The listing builds one solid part. Answer for the finished solid, in the listing's coordinates (mm). Coordinates: 2 decimals unless noted, no trailing zeros. Loops run counter-clockwise (first coordinate to the right, second up) from the corner with the lowest first, then second, coordinate; pieces in that order, holes last. Notation, with made-up numbers: (3, -9.5) - (15, -9.5) arc R8 cw to (15, -2.5) - close; hole circle Ø6 at (-22.5, 29). An arc over 180 degrees is marked (long way). One line per question, with ' | ' between items.
from build123d import *

# Parameters (mm, degrees)
F1_DEPTH = 254
F2_R     = 5.08
F3_R     = 11.0334695749
F3_R_2   = 10.3236193182
F3_R_3   = 10.3446634655
F4_DEPTH = 461.264


# Not quite as in the source:
# - the program builds the solid bodies; features that only make, move or delete a surface that nothing else refers to are left out


with BuildPart() as f1:
    # F0 (on Front) → F1 (new body)
    with BuildSketch(Plane.XZ):
        with BuildLine():
            ThreePointArc((-30.4000387615, -20.3651585358), (-24.0059784619, -10.8970905515), (-21.758691331, 0.3046065976))
            ThreePointArc((-21.758691331, 0.3046065976), (-23.9392938004, 11.3454431448), (-30.1536347581, 20.7282500411))
            ThreePointArc((-30.1536347581, 20.7282500411), (-36.5903525714, 0.2194028111), (-30.4000387615, -20.3651585358))
        make_face()
        with BuildLine():
            ThreePointArc((-30.1536347581, 20.7282500411), (-23.9392938004, 11.3454431448), (-21.758691331, 0.3046065976))
            ThreePointArc((-21.758691331, 0.3046065976), (-24.0059784619, -10.8970905515), (-30.4000387615, -20.3651585358))
            ThreePointArc((-30.4000387615, -20.3651585358), (-0.593995823, -36.5861887582), (29.7229129207, -21.3412859593))
            ThreePointArc((29.7229129207, -21.3412859593), (20.8050989976, 0), (29.7229129207, 21.3412859593))
            ThreePointArc((29.7229129207, 21.3412859593), (-0.3746112446, 36.5890927095), (-30.1536347581, 20.7282500411))
        make_face()
        with BuildLine():
            ThreePointArc((-30.4000387615, -20.3651585358), (-36.5903525714, 0.2194028111), (-30.1536347581, 20.7282500411))
            ThreePointArc((-30.1536347581, 20.7282500411), (-79.8407866027, 0.4787407551), (-30.4000387615, -20.3651585358))
        make_face()
        with BuildLine():
            ThreePointArc((36.5910103562, 0), (34.8316914131, 11.2096080304), (29.7229129207, 21.3412859593))
            ThreePointArc((29.7229129207, 21.3412859593), (20.8050989976, 0), (29.7229129207, -21.3412859593))
            ThreePointArc((29.7229129207, -21.3412859593), (34.8316914131, -11.2096080304), (36.5910103562, 0))
        make_face()
        with BuildLine():
            ThreePointArc((80.7949010024, 0), (62.364794546, 27.6757947177), (29.7229129207, 21.3412859593))
            ThreePointArc((29.7229129207, 21.3412859593), (34.8316914131, 11.2096080304), (36.5910103562, 0))
            ThreePointArc((36.5910103562, 0), (34.8316914131, -11.2096080304), (29.7229129207, -21.3412859593))
            ThreePointArc((29.7229129207, -21.3412859593), (62.364794546, -27.6757947177), (80.7949010024, 0))
        make_face()
    extrude(amount=F1_DEPTH)

    # F2
    f2_edges = [f1.edges().sort_by_distance(p)[0] for p in [
        (29.722913, -127, 21.341286),
        (-30.153635, -127, 20.72825),
        (29.722913, -127, -21.341286),
        (-30.400039, -127, -20.365159),
    ]]
    fillet(f2_edges, radius=F2_R)

    # F3 (on face) → F4 (cut)
    with BuildSketch(Plane.XZ.offset(254)):
        with Locations((-50.8, 0.3046065976)):
            Circle(F3_R)
        Circle(F3_R_2)
        with Locations((50.8, 0)):
            Circle(F3_R_3)
    extrude(amount=-F4_DEPTH, mode=Mode.SUBTRACT)


solid = f1.part
Item 1: Find the intervals of material crossed by line 1 (Z direction, x = 0, y = -197); line 2 (X direction, y = -38.5, z = -1); line 3 (X direction, y = -55.5, z = -5.5), in increasing order. Write a range as [from, to].
Taken from the geometry:
line 1: z = [-36.59, -10.32], [10.32, 36.59] | line 2: x = [-79.81, -61.76], [-39.84, -10.28], [10.28, 40.5], [61.1, 80.78] | line 3: x = [-79.26, -60.18], [-41.42, -8.74], [8.74, 42.04], [59.56, 80.29]
Item 2: Find section D-D, the plane y = -116.5. State how many separate pieces and enclosed holes the cut face has, plus the area to 3 significant figures.
Taken from the geometry:
separate pieces: 1 | enclosed holes: 3 | area: 7,770 mm2
Item 3: The mould has two halves that part along Z. Classify faces 1 (the face through (-1, 0, -16)), 2 (the face through (-0.96, -125.22, -36.58)), 3 (the face through (-2.238, -128.778, -10.078)): pulls with the +Z half, pulls with the -Z half, needs draft (parallel to the pull), parting line crosses it, or undercut.
Taken from the geometry:
face 1: needs draft | face 2: pulls with the -Z half | face 3: undercut
Item 4: Find section A-A, the plane x = 0. Write down the section's boundary in (y, z), plus the area to 3 significant figures.
Taken from the geometry:
outline: (-254, -36.59) - (0, -36.59) - (0, -10.32) - (-254, -10.32) - close; (-254, 10.32) - (0, 10.32) - (0, 36.59) - (-254, 36.59) - close | area: 13,300 mm2
Item 5: Find section C-C, the plane z = -20. Write down the section's boundary in (x, y), plus the area to 3 significant figures.
Taken from the geometry:
outline: (-71.56, -254) - (73.15, -254) - (73.15, 0) - (-71.56, 0) - close | area: 36,800 mm2
Item 6: Each of these flat-tipped pins is pushed along its axis until it touches: pin 1 Ø4 at (y, z) = (-227.5, 13) entering from -X; pin 2 Ø3 at (y, z) = (-57.5, 21.5) entering from +X; pin 3 Ø3 at (x, y) = (36.5, -147) entering from +Z; pin 4 Ø20 at (x, z) = (-50.8, 0.3) entering from -Y. Where does it stop, or does it pass through?
Taken from the geometry:
pin 1: stops at x = -77.8 | pin 2: stops at x = 73.15 | pin 3: stops at z = 27.13 | pin 4: passes through
Item 7: Find section B-B, the plane x = -50.8. Write down the section's boundary in (y, z).
Taken from the geometry:
outline: (-254, -28.74) - (0, -28.74) - (0, -10.73) - (-254, -10.73) - close; (-254, 11.34) - (0, 11.34) - (0, 29.35) - (-254, 29.35) - close
